The listing builds one solid part. Answer for the finished solid, in the listing's coordinates (mm). A direction names the side the tool comes from. Coordinates: 2 decimals unless noted, no trailing zeros. Loops run counter-clockwise (first coordinate to the right, second up) from the corner with the lowest first, then second, coordinate; pieces in that order, holes last. Notation, with made-up numbers: (82, 5.5) - (111, 5.5) arc R17 ccw to (111, 16.5) - close; hole circle Ø6 at (56.5, 19.5). An arc over 180 degrees is marked (long way). Write each question's results on one line, items separated by ' | '. Start each with the question number.
(1) For faces 1 (the cylindrical face through (0.86, -20.565, -3.874)), 2 (the flat face through (6.35, -13, 0)), determine the directions among +Z, -Z, +X, -X, +Y, -Y from which every point of the face is accessible in a straight line to the end or side of a thin tool.
(2) Find section B-B on y = -22.5. Determine the outline of the cut face in (x, z).
(3) Given pin 1 Ø1 at (x, y) = (3, -6) entering from +Z; pin 2 Ø8 at (y, z) = (1.5, -1) entering from +X; pin 3 Ø1 at (y, z) = (-5, 1) entering from -X, each flat-ended and moving along its own axis, determine where each tip first touches the part or whether it passes through.
(4) Find section C-C on y = -7. Determine the outline of the cut face in (x, z), then the cut area to 3 significant figures.
(5) Find section A-A on z = 0. Determine the outline of the cut face in (x, y).
(6) Consider line 1 (Y direction, x = 0.75, z = 5.25); line 2 (Y direction, x = 1, z = 2.5); line 3 (Z direction, x = 0, y = -19). Determine where each line is inside the solid, lowest interval first. Write a range as from..to.
(7) Determine the mould class of faces 3 (the flat face through (3.131, -13.215, 5.525)), 4 (the flat face through (-4, -12.1, -4)), 5 (the flat face through (4, -14.3, 2)), 6 (the conical face through (2.956, -7.18, 2.267)) for opening direction Y: released by +Y, released by -Y, zero draft, split by the parting line, or undercut.
Autodesk Inventor part; units mm, degrees
ref_plane "YZ Plane" through (0, 0, 0) normal (1, 0, 0) x (0, 1, 0)
ref_plane "XZ Plane" through (0, 0, 0) normal (0, 1, 0) x (-1, 0, 0)
ref_plane "XY Plane" through (0, 0, 0) normal (0, 0, 1) x (1, 0, 0)
sketch "Sketch1" plane through (0, 0, 0) normal (0, 0, 1) x (1, 0, 0)
  circle A0 centre (0, 0) radius 5
  line L0 (3.9688, -27) -> (-3.9687, -27)
  line L1 (-3.9687, -27) -> (-3.9687, 0)
  line L2 (-3.9687, 0) -> (3.9687, 0)
  line L3 (3.9687, 0) -> (3.9688, -27)
  line L4 (3.9688, -27) -> (-3.9687, 0) construction
  line L5 (-3.9687, -27) -> (3.9687, 0) construction
  line L6 (10, -14.3) -> (-10, -14.3)
  line L7 (-10, -14.3) -> (-10, -12.1)
  line L8 (-10, -12.1) -> (10, -12.1)
  line L9 (10, -12.1) -> (10, -14.3)
  line L10 (10, -14.3) -> (-10, -12.1) construction
  line L11 (-10, -14.3) -> (10, -12.1) construction
  line L12 (-5.0436, -12.1) -> (-2.8939, -4.0774)
  line L13 (2.8939, -4.0774) -> (5.0436, -12.1)
  line L14 (-5.0436, -12.1) -> (5.0436, -12.1) construction
  line L15 (0, 5) -> (0, -27)
  point P0 (0, -13.5)
  point P1 (0, -13.2)
  point P2 (-3.9688, -8.0887)
  point P3 (0, -12.1)
  point P4 (-3.9687, -14.3)
  dimension "d0" = 10
  dimension "d1" = 7.9375
  dimension "d2" = 32
  dimension "d3" = 20
  dimension "d4" = 12.7
  dimension "d5" = 30
  dimension "d6" = 2.2
revolve "Revolution1" add sketch "Sketch1" angle 360 about axis through (0, 5, 0) along (0, -1, 0) contours L15 L2 L1 A0 | L1 L2 L15 A0 | A0 L15 L8 L1 L12 | L1 L8 L12 | L8 L15 L6 L1 | L1 L6 L7 L8 | L6 L15 L0 L1
sketch "Sketch2" plane through (0, -14.3, 0) normal (0, -1, 0) x (1, 0, 0)
  circle A0 centre (0, 0) radius 2.8939
  line L0 (-6.35, 3.6662) -> (0, 7.3323)
  line L1 (0, 7.3323) -> (6.35, 3.6662)
  line L2 (6.35, 3.6662) -> (6.35, -3.6662)
  line L3 (6.35, -3.6662) -> (0, -7.3323)
  line L4 (0, -7.3323) -> (-6.35, -3.6662)
  line L5 (-6.35, -3.6662) -> (-6.35, 3.6662)
  circle A1 centre (0, 0) radius 3.9687
  circle A2 centre (0, 0) radius 10
  point P0 (0, 0)
  dimension "d8" = 12.7
extrude "Extrusion1" cut sketch "Sketch2" against normal through all contours A2
chamfer "Chamfer1" distance 0.25 angle 45 1 edges at (3.9688, -27, 0)
fillet "Fillet1" radius 0.25 1 edges at (3.9688, -14.3, 0)
fillet "Fillet2" radius 0.25 1 edges at (5.0436, -12.1, 0)
thread "Thread1"
properties part number "Gas Strut Ball Stud" material "Stainless Steel"
Values:
1) face 1: -Y | face 2: +Z, -Z, +X, +Y, -Y
2) outline: circle Ø7.94 at (0, 0)
3) pin 1: stops at z = 2.35 | pin 2: stops at x = 5 | pin 3: stops at x = -3.17
4) outline: circle Ø7.35 at (0, 0) | area: 42.5 mm²
5) outline: (-6.35, -14.3) - (-4.22, -14.3) arc R0.25 cw to (-3.97, -14.55) - (-3.97, -26.75) - (-3.72, -27) - (3.72, -27) - (3.97, -26.75) - (3.97, -14.55) arc R0.25 cw to (4.22, -14.3) - (6.35, -14.3) - (6.35, -12.1) - (5.24, -12.1) arc R0.25 cw to (4.99, -11.91) - (2.89, -4.08) arc R5 ccw (long way) to (-2.89, -4.08) - (-4.99, -11.91) arc R0.25 cw to (-5.24, -12.1) - (-6.35, -12.1) - close
6) line 1: y = -14.3..-12.1 | line 2: y = -27..4.21 | line 3: z = -3.97..3.97
7) face 3: zero draft | face 4: released by +Y | face 5: released by -Y | face 6: undercut
